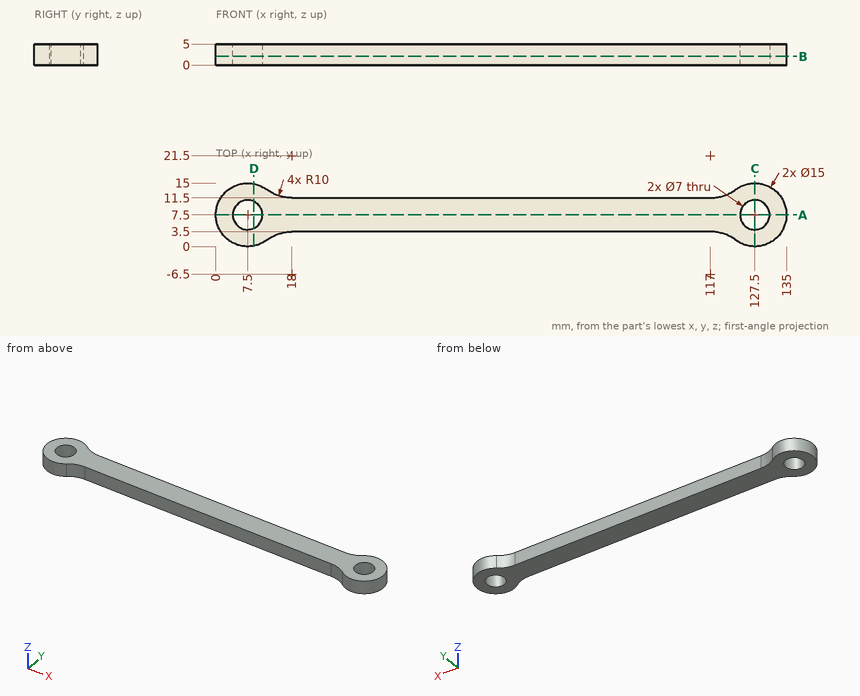
Could you check a few things on this drawing? It's one solid part, dimensions in mm from its lowest x, y, z. Round coordinates to 2 decimals unless told otherwise and drop trailing zeros. Loops run counter-clockwise (first coordinate to the right, second up) from the corner with the lowest first, then second, coordinate; pieces in that order, holes last. Notation, with made-up numbers: M 26.5,83 L 47.5,83 A17 cw 47.5,108 Z; hole C 32,37.5 d11. An arc over 180 degrees is marked long. Write each question's results on one line, items separated by ' | '. Start each with the question number.
(1) I want a section at C-C (x = 127.5). Please give me the cut outline in (y, z), then the cut area to 3 significant figures.
(2) I want a section at B-B (z = 2.05). Please give me the cut outline in (x, y), then the cut area to 3 significant figures.
(3) I want a section at A-A (y = 7.5). Please give me the cut outline in (x, z), then the cut area to 3 significant figures.
(4) If I drill on probe 1 along X at (y, z) = (7.5, 2.2); probe 2 along X at (y, z) = (9.75, 4.6); probe 3 along Y at (x, z) = (7.5, 2.8), over which ranges is the centre line in solid material (lowest first)? Write a range as from..to.
(5) Will these pins go through, and if not, where does the flat tip stop? P1, Ø4, axis at x = 7.5, y = 7.5, coming from the +Z side; P2, Ø1, axis at y = 1.5, z = 3.5, coming from the -X side; P3, Ø1.5, axis at x = 79, z = 3, coming from the -Y side; P4, Ø1.5, axis at y = 3, z = 1.5, coming from the -X side.
(6) I want a section at D-D (x = 9). Please give me the cut outline in (y, z).
Solved:
1) outline: M 0,0 L 4,0 L 4,5 L 0,5 Z; M 11,0 L 15,0 L 15,5 L 11,5 Z | area: 40.0 mm²
2) outline: M 12,1.5 A10 cw 18,3.5 L 117,3.5 A10 cw 123,1.5 A7.5 ccw long 123,13.5 A10 cw 117,11.5 L 18,11.5 A10 cw 12,13.5 A7.5 ccw long Z; hole C 7.5,7.5 d7; hole C 127.5,7.5 d7 | area: 1,130 mm²
3) outline: M 0,0 L 4,0 L 4,5 L 0,5 Z; M 11,0 L 124,0 L 124,5 L 11,5 Z; M 131,0 L 135,0 L 135,5 L 131,5 Z | area: 605 mm²
4) probe 1: x = 0..4, 11..124, 131..135 | probe 2: x = 0.35..4.82, 10.18..124.82, 130.18..134.65 | probe 3: y = 0..4, 11..15
5) P1: passes through | P2: stops at x = 2.4 | P3: stops at y = 3.5 | P4: stops at x = 1
6) outline: M 0.15,0 L 4.34,0 L 4.34,5 L 0.15,5 Z; M 10.66,0 L 14.85,0 L 14.85,5 L 10.66,5 Z
